The listing builds one solid part. Answer for the finished solid, in the listing's coordinates (mm). Coordinates: 2 decimals unless noted, no trailing zeros. Write each loop counter-clockwise with the first axis right and the second up, starting at its lowest first coordinate (ties: lowest second). Pieces come first, ordered by that corner, then holes.
(1) Straight lines are drawn through the part: line 1 (Z direction, x = 0, y = -2.4); line 2 (X direction, y = 19.5, z = 5); line 3 (Z direction, x = 46, y = 17.25). For each, find the intervals that lie inside material, in ascending order.
(2) The part is cut by section A-A on y = 9. Determine the outline of the cut face in (x, z).
(3) Given P1, Ø5, axis at x = 59, y = 14, coming from the -Z side; P2, Ø4, axis at x = 72.5, z = 4, coming from the -Y side; P3, Ø1.6, axis at x = -80, y = 21, coming from the +Z side; P4, Ø12, axis at x = 65.5, y = 19, coming from the +Z side, each flat-ended and moving along its own axis, determine where each tip first touches the part or whether it passes through.
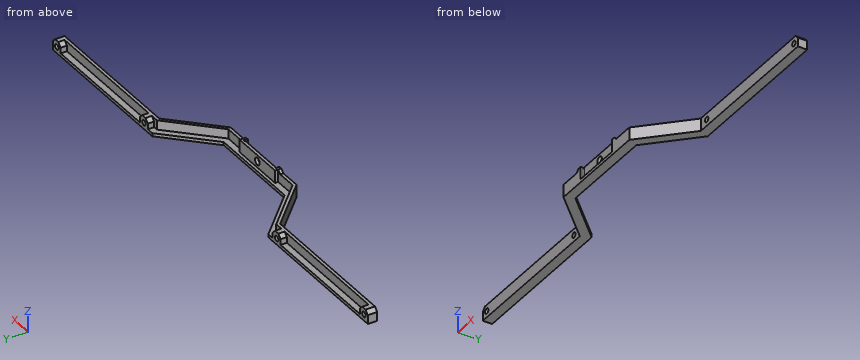
from build123d import *

# Parameters (mm, degrees)
F1_DEPTH  = 1.5875
F3_DEPTH  = 4.7625
F4_W      = 6.35
F4_H      = 6.35
F5_DEPTH  = 3.175
F6_SIZE   = 1.8598642
F7_W      = 28.575
F7_H      = 3.175
F8_DEPTH  = 1.5875
F9_W      = 25.4
F9_H      = 1.5875
F10_DEPTH = 6.35
F11_SIZE  = 1.58749
F12_R     = 1.35255
F12_R_2   = 1.8288
F13_DEPTH = 25.4
F14_R     = 0.396875
F15_DEPTH = 6.35


# Not quite as in the source:
# - a fillet or chamfer is up to 0.001 mm smaller than in the source, because OpenCascade refuses the exact size


with BuildPart() as f1:
    # F0 (on Top) → F1 (new body)
    with BuildSketch(Plane.XY):
        Polygon((-46.7826079092, 22.225), (-127, 22.225), (-127, 17.4625), (-48.7553, 17.4625), (-26.5303, -4.7625), (26.5303, -4.7625), (48.7553, 17.4625), (127, 17.4625), (127, 22.225), (46.7826079092, 22.225), (24.5576079092, 0), (-24.5576079092, 0), align=None)
    extrude(amount=F1_DEPTH)

    # F2 (on face) → F3 (join)
    with BuildSketch(Plane.XY.offset(1.5875)):
        Polygon((-127, 19.05), (-127, 17.4625), (-48.7553, 17.4625), (-26.5303, -4.7625), (26.5303, -4.7625), (48.7553, 17.4625), (127, 17.4625), (127, 19.05), (48.0977359697, 19.05), (25.8727359697, -3.175), (14.2875, -3.175), (14.2875, -1.5875), (-14.2875, -1.5875), (-14.2875, -3.175), (-25.8727359697, -3.175), (-48.0977359697, 19.05), align=None)
    extrude(amount=F3_DEPTH)

    # F4 (on face) → F5 (join, through all)
    with BuildSketch(Plane(origin=(0, 19.05, 0), x_dir=(-1, 0, 0), z_dir=(0, 1, 0))):
        with Locations((-53.5178, 3.175)):
            Rectangle(F4_W, F4_H)
        with Locations((-123.825, 3.175)):
            Rectangle(F4_W, F4_H)
        with Locations((123.825, 3.175)):
            Rectangle(F4_W, F4_H)
        with Locations((53.5178, 3.175)):
            Rectangle(F4_W, F4_H)
    extrude(amount=F5_DEPTH)

    # F6
    f6_edges = [f1.edges().sort_by_distance(p)[0] for p in [
        (-127, 19.84375, 6.35),
        (-120.65, 20.6375, 6.35),
        (-56.6928, 20.6375, 6.35),
        (-50.3428, 20.6375, 6.35),
        (50.3428, 20.6375, 6.35),
        (56.6928, 20.6375, 6.35),
        (120.65, 20.6375, 6.35),
        (127, 19.84375, 6.35),
    ]]
    chamfer(f6_edges, length=F6_SIZE)

    # F7 (on face) → F8 (join)
    with BuildSketch(Plane.XY.offset(6.35)):
        with Locations((0, -3.175)):
            Rectangle(F7_W, F7_H)
    extrude(amount=F8_DEPTH)

    # F9 (on face) → F10 (cut, through all)
    with BuildSketch(Plane.XY.offset(7.9375)):
        with Locations((0, -3.96875)):
            Rectangle(F9_W, F9_H)
    extrude(amount=-F10_DEPTH, mode=Mode.SUBTRACT)

    # F11 (size 1.5875 in the source; OpenCascade refuses exactly that, so slightly less here)
    f11_edges = [f1.edges().sort_by_distance(p)[0] for p in [
        (-14.2875, -3.96875, 6.35),
        (14.2875, -3.96875, 6.35),
    ]]
    chamfer(f11_edges, length=F11_SIZE)

    # F12 (on face) → F13 (cut, through all)
    with BuildSketch(Plane.XZ.offset(3.175)):
        with Locations((53.5178, 3.175)):
            Circle(F12_R)
        with Locations((123.825, 3.175)):
            Circle(F12_R)
        with Locations((-123.825, 3.175)):
            Circle(F12_R)
        with Locations((-53.5178, 3.175)):
            Circle(F12_R)
        with Locations((0, 4.7625)):
            Circle(F12_R_2)
    extrude(amount=-F13_DEPTH, mode=Mode.SUBTRACT)

    # F14 (on face) → F15 (cut, through all)
    with BuildSketch(Plane.XY.offset(7.9375)):
        with Locations((12.7, -3.175)):
            Circle(F14_R)
        with Locations((-12.7, -3.175)):
            Circle(F14_R)
    extrude(amount=-F15_DEPTH, mode=Mode.SUBTRACT)


solid = f1.part
Model answer:
1. line 1: z = 0 to 2.93, 6.59 to 7.94
1. line 2: x = -126.49 to -121.16, -56.18 to -50.85, 50.85 to 56.18, 121.16 to 126.49
1. line 3: z = 0 to 1.59
2. outline: (-40.29, 0) - (-33.56, 0) - (-33.56, 1.59) - (-38.05, 1.59) - (-38.05, 6.35) - (-40.29, 6.35) - close; (33.56, 0) - (40.29, 0) - (40.29, 6.35) - (38.05, 6.35) - (38.05, 1.59) - (33.56, 1.59) - close
3. P1: passes through
3. P2: stops at y = 17.46
3. P3: stops at z = 1.59
3. P4: stops at z = 6.35
